```python
from build123d import *

# Parameters (mm, degrees)
EXTRUDE_1_DEPTH = 4


with BuildPart() as part:
    # 草图1 → 凸台-拉伸1 (new body)
    with BuildSketch(Plane.XY):
        with BuildLine():
            Line((-4.5, 34), (-4.5, 0))
            ThreePointArc((-4.5, 0), (0, -4.5), (4.5, 0))
            Line((4.5, 0), (4.5, 34))
            ThreePointArc((4.5, 34), (0, 38.5), (-4.5, 34))
        make_face()
        with BuildLine():
            Line((-3, 34), (-3, 6))
            ThreePointArc((-3, 6), (-2.4, 5.4), (-1.8, 6))
            Line((-1.8, 6), (-1.8, 30.750384638))
            ThreePointArc((-1.8, 30.750384638), (-1.580305955, 31.164423974), (-1.114285714, 31.214615404))
            ThreePointArc((-1.114285714, 31.214615404), (2.484236014, 35.681835732), (-3, 34))
        make_face(mode=Mode.SUBTRACT)
        with BuildLine():
            Line((3, 0), (3, 28))
            ThreePointArc((3, 28), (2.4, 28.6), (1.8, 28))
            Line((1.8, 28), (1.8, 3.249615362))
            ThreePointArc((1.8, 3.249615362), (1.580305955, 2.835576026), (1.114285714, 2.785384596))
            ThreePointArc((1.114285714, 2.785384596), (-2.484236014, -1.681835732), (3, 0))
        make_face(mode=Mode.SUBTRACT)
    extrude(amount=EXTRUDE_1_DEPTH)


solid = part.part
```
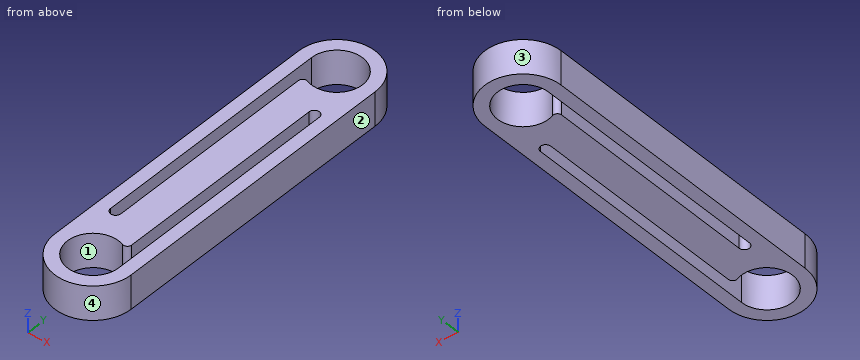
Build history of the part. All positions in model axes, mm. Face numbers are marked on the shaded views. Round coordinates to 2 decimals unless told otherwise and drop trailing zeros. Order: outer loops, then holes, each group sorted by start corner. A loop starts at its lowest first (then second) coordinate and runs counter-clockwise, first axis right, second up. Notation, with made-up numbers: (76, 60) -> (129, 60) arc R18 cw to (129, 85) -> close; hole circle Ø8 at (8, 80). An arc over 180 degrees is marked (long way). Answer in a Markdown table with one row per item.
1) Band-saw the part on D-D on z = 1.65. Give the cut face in (x, y).
Values:
| item | result |
|---|---|
| outline | (-4.5, 0) arc R4.5 ccw to (4.5, 0) -> (4.5, 34) arc R4.5 ccw to (-4.5, 34) -> close; hole (-3, 6) arc R0.6 ccw to (-1.8, 6) -> (-1.8, 30.75) arc R0.5 cw to (-1.11, 31.21) arc R3 ccw (long way) to (-3, 34) -> close; hole (1.11, 2.79) arc R3 ccw (long way) to (3, 0) -> (3, 28) arc R0.6 ccw to (1.8, 28) -> (1.8, 3.25) arc R0.5 cw to start |
2) Wall check: L1, parallel to X at y = 7, z = 1.2; L2, parallel to Y at x = 0, z = 2.8; L3, parallel to X at y = 4, z = 0.3. Give the ranges that are in metal, low to high.
Values:
| item | result |
|---|---|
| L1 | -4.5 to -3, -1.8 to 1.8, 3 to 4.5 |
| L2 | -4.5 to -3, 3 to 31, 37 to 38.5 |
| L3 | -4.5 to 1.8, 3 to 4.5 |
3) Mould opens along Y. For the marked faces 1, 2, 3 and 4 say: released by +Y, released by -Y, zero draft, split by the parting line, or undercut.
Values:
| item | result |
|---|---|
| face 1 | undercut |
| face 2 | zero draft |
| face 3 | released by +Y |
| face 4 | released by -Y |
4) Band-saw the part on A-A on x = 0. Give the cut face in (y, z).
Values:
| item | result |
|---|---|
| outline | (-4.5, 0) -> (-3, 0) -> (-3, 4) -> (-4.5, 4) -> close; (3, 0) -> (31, 0) -> (31, 4) -> (3, 4) -> close; (37, 0) -> (38.5, 0) -> (38.5, 4) -> (37, 4) -> close |
5) Band-saw the part on B-B on y = 30. Give the cut face in (x, z).
Values:
| item | result |
|---|---|
| outline | (-4.5, 0) -> (-3, 0) -> (-3, 4) -> (-4.5, 4) -> close; (-1.8, 0) -> (4.5, 0) -> (4.5, 4) -> (-1.8, 4) -> close |
6) Band-saw the part on C-C on y = 8. Give the cut face in (x, z).
Values:
| item | result |
|---|---|
| outline | (-4.5, 0) -> (-3, 0) -> (-3, 4) -> (-4.5, 4) -> close; (-1.8, 0) -> (1.8, 0) -> (1.8, 4) -> (-1.8, 4) -> close; (3, 0) -> (4.5, 0) -> (4.5, 4) -> (3, 4) -> close |
